Here's how the part is built. I have some questions about the finished solid (model axes, mm). Face numbers are marked on the shaded views. A direction names the side the tool comes from. Round coordinates to 2 decimals unless told otherwise and drop trailing zeros. Loops run counter-clockwise (first coordinate to the right, second up) from the corner with the lowest first, then second, coordinate; pieces in that order, holes last. Notation, with made-up numbers: M -5,64.5 L 54,64.5 A9 ccw 54,77.5 Z; hole C 82.5,-5 d6. An arc over 180 degrees is marked long. Answer as a JSON object with one key per item and string values.
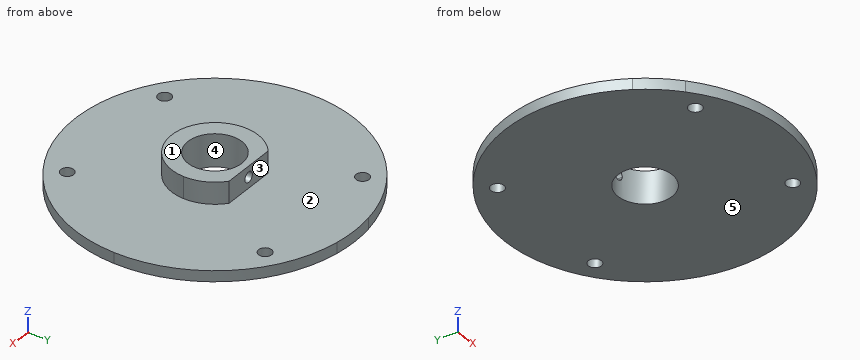
from build123d import *

# Parameters (mm, degrees)
SKETCH_1_R          = 5
SKETCH_1_R_2        = 1.2
EXTRUDE_1_DEPTH     = 2
SKETCH_2_R          = 5
EXTRUDE_2_DEPTH     = 4
CUT_EXTRUDE_1_DEPTH = 4


with BuildPart() as part:
    # 草图1 → 凸台-拉伸1 (new body)
    # profile 1 of 9: a face of its own
    with BuildSketch(Plane.XY):
        with BuildLine():
            Line((50.787618615, 13.919461135), (48.798857294, 18.312980654))
            ThreePointArc((48.798857294, 18.312980654), (40.538542245, 4), (43.589554969, -12.241475957))
            ThreePointArc((43.589554969, -12.241475957), (45.937273528, -15.497674419), (48.798857294, -18.312980654))
            Line((48.798857294, -18.312980654), (53.988393324, -6.848393324))
            Line((53.988393324, -6.848393324), (54.3, -7.16))
            Line((54.3, -7.16), (54.3, -21.733614518))
            ThreePointArc((54.3, -21.733614518), (64, -23.8), (73.7, -21.733614518))
            Line((73.7, -21.733614518), (73.7, -6.915634891))
            Line((73.7, -6.915634891), (74.1123773, -7.071013151))
            Line((74.1123773, -7.071013151), (79.201142706, -18.312980654))
            ThreePointArc((79.201142706, -18.312980654), (85.543295899, -10.115651328), (87.8, 0))
            ThreePointArc((87.8, 0), (85.543295899, 10.115651328), (79.201142706, 18.312980654))
            Line((79.201142706, 18.312980654), (76.899825635, 13.228971143))
            Line((76.899825635, 13.228971143), (73.7, 14.677397496))
            Line((73.7, 14.677397496), (73.7, 21.733614518))
            ThreePointArc((73.7, 21.733614518), (70.904263941, 22.776548014), (68, 23.461457755))
            ThreePointArc((68, 23.461457755), (64, 23.8), (60, 23.461457755))
            ThreePointArc((60, 23.461457755), (57.095736059, 22.776548014), (54.3, 21.733614518))
            Line((54.3, 21.733614518), (54.3, 13.919461135))
            Line((54.3, 13.919461135), (50.787618615, 13.919461135))
        make_face()
        with Locations((64, 0)):
            Circle(SKETCH_1_R, mode=Mode.SUBTRACT)
    # profile 2 of 9: a face of its own
    with BuildSketch(Plane.XY):
        with BuildLine():
            ThreePointArc((43.589554969, -12.241475957), (40.538542245, 4), (48.798857294, 18.312980654))
            ThreePointArc((48.798857294, 18.312980654), (51.432505778, 20.211335655), (54.3, 21.733614518))
            ThreePointArc((54.3, 21.733614518), (57.095736059, 22.776548014), (60, 23.461457755))
            Line((60, 23.461457755), (60, 25.488036409))
            ThreePointArc((60, 25.488036409), (40.557730485, 10.774970998), (42.051507242, -13.561108569))
            Line((42.051507242, -13.561108569), (43.589554969, -12.241475957))
        make_face()
    # profile 3 of 9: a face of its own
    with BuildSketch(Plane.XY):
        with BuildLine():
            ThreePointArc((54.3, -21.733614518), (51.432505778, -20.211335655), (48.798857294, -18.312980654))
            Line((48.798857294, -18.312980654), (47.260809567, -19.632613266))
            ThreePointArc((47.260809567, -19.632613266), (74.811310902, -23.425532152), (89.8, 0))
            ThreePointArc((89.8, 0), (83.606631531, 16.76961538), (68, 25.488036409))
            Line((68, 25.488036409), (68, 23.461457755))
            ThreePointArc((68, 23.461457755), (70.904263941, 22.776548014), (73.7, 21.733614518))
            ThreePointArc((73.7, 21.733614518), (76.567494222, 20.211335655), (79.201142706, 18.312980654))
            ThreePointArc((79.201142706, 18.312980654), (85.543295899, 10.115651328), (87.8, 0))
            ThreePointArc((87.8, 0), (85.543295899, -10.115651328), (79.201142706, -18.312980654))
            ThreePointArc((79.201142706, -18.312980654), (76.567494222, -20.211335655), (73.7, -21.733614518))
            ThreePointArc((73.7, -21.733614518), (64, -23.8), (54.3, -21.733614518))
        make_face()
    # profile 4 of 9: a face of its own
    with BuildSketch(Plane.XY):
        with BuildLine():
            Line((60, 25.488036409), (60, 23.461457755))
            ThreePointArc((60, 23.461457755), (64, 23.8), (68, 23.461457755))
            Line((68, 23.461457755), (68, 25.488036409))
            ThreePointArc((68, 25.488036409), (64, 25.8), (60, 25.488036409))
        make_face()
    # profile 5 of 9: a face of its own
    with BuildSketch(Plane.XY):
        with BuildLine():
            ThreePointArc((48.798857294, -18.312980654), (45.937273528, -15.497674419), (43.589554969, -12.241475957))
            Line((43.589554969, -12.241475957), (42.051507242, -13.561108569))
            ThreePointArc((42.051507242, -13.561108569), (44.419397354, -16.8), (47.260809567, -19.632613266))
            Line((47.260809567, -19.632613266), (48.798857294, -18.312980654))
        make_face()
    # profile 6 of 9: a face of its own
    with BuildSketch(Plane.XY):
        with BuildLine():
            Line((53.988393324, -6.848393324), (48.798857294, -18.312980654))
            ThreePointArc((48.798857294, -18.312980654), (51.432505778, -20.211335655), (54.3, -21.733614518))
            Line((54.3, -21.733614518), (54.3, -7.16))
            Line((54.3, -7.16), (53.988393324, -6.848393324))
        make_face()
        with Locations((51.549428647, -18.312980654)):
            Circle(SKETCH_1_R_2, mode=Mode.SUBTRACT)
    # profile 7 of 9: a face of its own
    with BuildSketch(Plane.XY):
        with BuildLine():
            Line((73.7, -6.915634891), (73.7, -21.733614518))
            ThreePointArc((73.7, -21.733614518), (76.567494222, -20.211335655), (79.201142706, -18.312980654))
            Line((79.201142706, -18.312980654), (74.1123773, -7.071013151))
            Line((74.1123773, -7.071013151), (73.7, -6.915634891))
        make_face()
        with Locations((76.450571353, -18.312980654)):
            Circle(SKETCH_1_R_2, mode=Mode.SUBTRACT)
    # profile 8 of 9: a face of its own
    with BuildSketch(Plane.XY):
        with BuildLine():
            ThreePointArc((79.201142706, 18.312980654), (76.567494222, 20.211335655), (73.7, 21.733614518))
            Line((73.7, 21.733614518), (73.7, 14.677397496))
            Line((73.7, 14.677397496), (76.899825635, 13.228971143))
            Line((76.899825635, 13.228971143), (79.201142706, 18.312980654))
        make_face()
        with Locations((76.450571353, 18.312980654)):
            Circle(SKETCH_1_R_2, mode=Mode.SUBTRACT)
    # profile 9 of 9: a face of its own
    with BuildSketch(Plane.XY):
        with BuildLine():
            ThreePointArc((54.3, 21.733614518), (51.432505778, 20.211335655), (48.798857294, 18.312980654))
            Line((48.798857294, 18.312980654), (50.787618615, 13.919461135))
            Line((50.787618615, 13.919461135), (54.3, 13.919461135))
            Line((54.3, 13.919461135), (54.3, 21.733614518))
        make_face()
        with Locations((51.549428647, 18.312980654)):
            Circle(SKETCH_1_R_2, mode=Mode.SUBTRACT)
    extrude(amount=EXTRUDE_1_DEPTH)

    # 草图2 → 凸台-拉伸2 (add)
    with BuildSketch(Plane.XY.offset(2)):
        with BuildLine():
            ThreePointArc((72, 0), (71.211102551, 3.464101615), (69, 6.244997998))
            Line((69, 6.244997998), (59, 6.244997998))
            ThreePointArc((59, 6.244997998), (60.535898385, -7.211102551), (72, 0))
        make_face()
        with Locations((64, 0)):
            Circle(SKETCH_2_R, mode=Mode.SUBTRACT)
    extrude(amount=EXTRUDE_2_DEPTH)

    # 草图3 → 切除-拉伸1 (cut)
    with BuildSketch(Plane(origin=(0, 6.244997998, 0), x_dir=(1, 0, 0), z_dir=(0, 1, 0))):
        with BuildLine():
            ThreePointArc((64.95, -4), (64.932858567, -3.820347855), (64.882052856, -3.647178857))
            Line((64.882052856, -3.647178857), (63.117947144, -4.352821143))
            ThreePointArc((63.117947144, -4.352821143), (64.179652145, -4.932858567), (64.95, -4))
        make_face()
        with BuildLine():
            Line((63.117947144, -4.352821143), (64.882052856, -3.647178857))
            ThreePointArc((64.882052856, -3.647178857), (63.647178857, -3.117947144), (63.117947144, -4.352821143))
        make_face()
    extrude(amount=-CUT_EXTRUDE_1_DEPTH, mode=Mode.SUBTRACT)


solid = part.part
Item 1: I want a section at C-C, the plane z = 1. Please give me the cut outline in (x, y).
Resolved:
{"outline": "C 64,0 d51.6; hole C 51.55,-18.31 d2.4; hole C 51.55,18.31 d2.4; hole C 64,0 d10; hole C 76.45,-18.31 d2.4; hole C 76.45,18.31 d2.4"}
Item 2: I'm going to push flat-ended pins straight in: pin 1 Ø8 at (x, y) = (82.5, 6.5) entering from +Z; pin 2 Ø1.5 at (y, z) = (10.5, 1.5) entering from +X; pin 3 Ø2 at (y, z) = (1.5, 0.5) entering from +X. Where does each tip first touch, or does it pass through?
Resolved:
{"pin 1": "z = 2", "pin 2": "x = 87.89", "pin 3": "x = 89.8"}
Item 3: On a 3-axis mill with a long thin cutter (end or side, diameter ignored), from which of +Z, -Z, +X, -X, +Y, -Y can I reach the whole of each face in a straight line? I mean the marked faces 1, 2 and 3. Say none if no direction works.
Resolved:
{"face 1": "+Z, +X, -X, +Y, -Y", "face 2": "+Z", "face 3": "+Z, +X, -X, +Y"}
Item 4: I want a section at B-B, the plane y = -3. Please give me the cut outline in (x, z).
Resolved:
{"outline": "M 38.38,0 L 60,0 L 60,6 L 56.58,6 L 56.58,2 L 38.38,2 Z; M 68,0 L 89.62,0 L 89.62,2 L 71.42,2 L 71.42,6 L 68,6 Z"}
Item 5: I want a section at A-A, the plane x = 64. Please give me the cut outline in (y, z) (3 decimals).
Resolved:
{"outline": "M -25.8,0 L -5,0 L -5,6 L -8,6 L -8,2 L -25.8,2 Z; M 5,0 L 25.8,0 L 25.8,2 L 6.245,2 L 6.245,3.05 L 5,3.05 Z; M 5,4.95 L 6.245,4.95 L 6.245,6 L 5,6 Z"}
Item 6: I want a section at D-D, the plane x = 77. Please give me the cut outline in (y, z), then the cut area to 3 significant figures.
Resolved:
{"outline": "M -22.29,0 L -19.38,0 L -19.38,2 L -22.29,2 Z; M -17.25,0 L 17.25,0 L 17.25,2 L -17.25,2 Z; M 19.38,0 L 22.29,0 L 22.29,2 L 19.38,2 Z", "area": "80.6 mm²"}
Item 7: Please list where these lines run through material, in increasing order: probe 1 along Z at (x, y) = (68, -22); probe 2 along X at (y, z) = (2, 3.25); probe 3 along X at (y, z) = (-10, 1). Write a range as from..to.
Resolved:
{"probe 1": "0..2", "probe 2": "56.25..59.42, 68.58..71.75", "probe 3": "40.22..87.78"}
Item 8: If we mould it in two halves opening along X, with no side actions, what happens to the marked faces 4 and 5? For each: pulls with the +X half, pulls with the -X half, needs draft (parallel to the pull), parting line crosses it, or undercut.
Resolved:
{"face 4": "undercut", "face 5": "needs draft"}
